Verification items for the finished model (mm, model axes). Face numbers are marked on the shaded views. Give positions to 0.01 mm unless a question says otherwise; leave off trailing zeros. Write each loop counter-clockwise with the first axis right and the second up, starting at its lowest first coordinate (ties: lowest second). Pieces come first, ordered by that corner, then holes. Notation, with made-up numbers: (-14.75, 9.25) - (43.25, 9.25) arc R23 ccw to (43.25, 27.25) - close; hole circle Ø5 at (-25.5, 79). An arc over 180 degrees is marked (long way). Answer as a JSON object with one key per item and string values. Group by question number.
Item 1: Go/stop test with flat-tipped pins: pin 1 (0.8 mm diameter, centred on x = 20.5, y = 30.5, fed in from +Z); pin 2 (3.5 mm diameter, centred on x = 32, z = 11.5, fed in from +Y); pin 3 (1 mm diameter, centred on x = 25, y = 14.5, fed in from +Z); pin 4 (10 mm diameter, centred on x = 29, z = 10.5, fed in from +Y). Record where each tip stops, or that it passes through.
Item 2: Sectioned sample at A-A, the plane x = 22. Record the boundary of the cut face in (y, z).
Item 3: Sectioned sample at B-B, the plane y = 14.5. Record the boundary of the cut face in (x, z), and give its area (3 significant figures).
Item 4: Sectioned sample at C-C, the plane z = 25.5. Record the boundary of the cut face in (x, y).
Item 5: Scan lines: line 1 along X through (y, z) = (11, 4.75); line 2 along X through (y, z) = (23.5, 20.5); line 3 along Y through (x, z) = (18.5, 23). Record each from-to range of solid material in increasing order. Write a range as [from, to].
Item 6: Draft check along X on the marked faces 1, 2 and 3. Enter one of: +X half, -X half, draft (parallel to the pull), parting line (faces both ways), or undercut.
```python
from build123d import *

# Parameters (mm, degrees)
SKETCH2_W           = 50.8
SKETCH2_H           = 31.75
BOSS_EXTRUDE1_DEPTH = 27.94
CUT_EXTRUDE2_DEPTH  = 27.94
FILLET1_R           = 7.62
SKETCH5_W           = 1.27
SKETCH5_H           = 0.685488516
BOSS_EXTRUDE2_DEPTH = 27.94
SKETCH6_W           = 0.849135511
SKETCH6_H           = 0.685488516
BOSS_EXTRUDE3_DEPTH = 25.4
FILLET2_R           = 2.54
FILLET3_R           = 2.54


with BuildPart() as part:
    # Sketch2 → Boss-Extrude1 (new body)
    with BuildSketch(Plane.XY):
        with Locations((25.4, 15.875)):
            Rectangle(SKETCH2_W, SKETCH2_H)
    extrude(amount=BOSS_EXTRUDE1_DEPTH)

    # Sketch3 → Cut-Extrude2 (cut)
    with BuildSketch(Plane.XY.offset(27.94)):
        Polygon((24.154806831, 18.987982921), (24.154806831, 8.376771572), (35.415684182, 8.376771572), (35.415684182, 18.987982921), (35.415684182, 31.75), (12.893929481, 31.75), (12.893929481, 18.987982921), align=None)
    extrude(amount=-CUT_EXTRUDE2_DEPTH, mode=Mode.SUBTRACT)

    # Fillet1
    fillet1_edges = [part.edges().sort_by_distance(p)[0] for p in [
        (50.8, 31.75, 13.97),
    ]]
    fillet(fillet1_edges, radius=FILLET1_R)

    # Sketch5 → Boss-Extrude2 (add)
    with BuildSketch(Plane.ZY.offset(-35.415684182)):
        with Locations((0.724212181, 30.851974388)):
            Rectangle(SKETCH5_W, SKETCH5_H)
        with Locations((27.068073402, 30.851974388)):
            Rectangle(SKETCH5_W, SKETCH5_H)
    extrude(amount=BOSS_EXTRUDE2_DEPTH)

    # Sketch6 → Boss-Extrude3 (add)
    with BuildSketch(Plane.XY.offset(1.359212181)):
        with Locations((27.792387074, 30.851974388)):
            Rectangle(SKETCH6_W, SKETCH6_H)
    extrude(amount=BOSS_EXTRUDE3_DEPTH)

    # Fillet2
    fillet2_edges = [part.edges().sort_by_distance(p)[0] for p in [
        (50.8, 0, 13.97),
    ]]
    fillet(fillet2_edges, radius=FILLET2_R)

    # Fillet3
    fillet3_edges = [part.edges().sort_by_distance(p)[0] for p in [
        (0, 0, 13.97),
    ]]
    fillet(fillet3_edges, radius=FILLET3_R)


solid = part.part
```
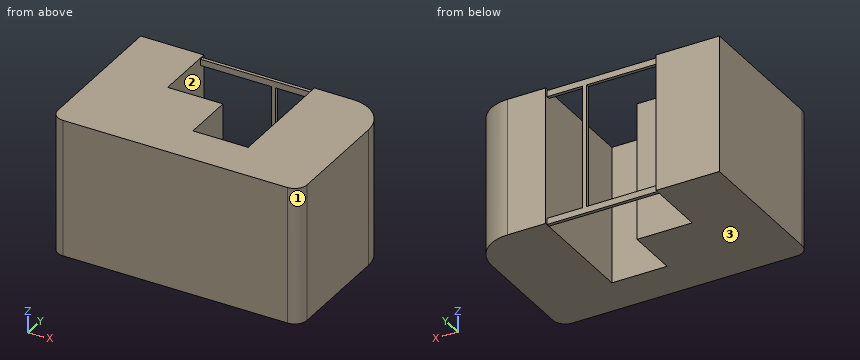
Geometry check:
{
 "1": {"pin 1": "z = 27.7", "pin 2": "y = 8.38", "pin 3": "through", "pin 4": "y = 31.19"},
 "2": {"outline": "(0, 0) - (18.99, 0) - (18.99, 27.94) - (0, 27.94) - close; (30.51, 0.09) - (31.19, 0.09) - (31.19, 1.36) - (30.51, 1.36) - close; (30.51, 26.43) - (31.19, 26.43) - (31.19, 27.7) - (30.51, 27.7) - close"},
 "3": {"outline": "(0, 0) - (24.15, 0) - (24.15, 27.94) - (0, 27.94) - close; (35.42, 0) - (50.8, 0) - (50.8, 27.94) - (35.42, 27.94) - close", "area": "1,100 mm^2"},
 "4": {"outline": "(0, 2.54) arc R2.54 ccw to (2.54, 0) - (48.26, 0) arc R2.54 ccw to (50.8, 2.54) - (50.8, 24.13) arc R7.62 ccw to (43.18, 31.75) - (35.42, 31.75) - (35.42, 8.38) - (24.15, 8.38) - (24.15, 18.99) - (12.89, 18.99) - (12.89, 31.75) - (0, 31.75) - close; (27.37, 30.51) - (28.22, 30.51) - (28.22, 31.19) - (27.37, 31.19) - close"},
 "5": {"line 1": "[0, 24.15], [35.42, 50.8]", "line 2": "[0, 12.89], [35.42, 50.8]", "line 3": "[0, 18.99]"},
 "6": {"face 1": "+X half", "face 2": "undercut", "face 3": "draft"}
}
